from build123d import *

# Parameters (mm, degrees)
F0_W     = 304.8
F0_H     = 381
F1_DEPTH = 355.6
F2_R     = 25.4
F3_R     = 127
F4_DEPTH = 152.4


with BuildPart() as f1:
    # F0 (on Front) → F1 (new body)
    with BuildSketch(Plane.XZ):
        Rectangle(F0_W, F0_H)
    extrude(amount=F1_DEPTH)

    # F2
    f2_edges = [f1.edges().sort_by_distance(p)[0] for p in [
        (-152.4, -355.6, 0),
        (0, -355.6, 190.5),
        (152.4, -355.6, 0),
        (0, -355.6, -190.5),
        (-152.4, -177.8, -190.5),
        (-152.4, -177.8, 190.5),
        (152.4, -177.8, 190.5),
        (152.4, -177.8, -190.5),
        (0, 0, -190.5),
        (152.4, 0, 0),
        (0, 0, 190.5),
        (-152.4, 0, 0),
    ]]
    fillet(f2_edges, radius=F2_R)

    # F3 (on face) → F4 (join)
    with BuildSketch(Plane(origin=(0, 0, 0), x_dir=(-1, 0, 0), z_dir=(0, 1, 0))):
        Circle(F3_R)
    extrude(amount=F4_DEPTH)


solid = f1.part
The model under review builds one solid part; all positions refer to its coordinate system, in mm. A direction names the side the tool comes from. Coordinates: 2 decimals unless noted, no trailing zeros. Write each loop counter-clockwise with the first axis right and the second up, starting at its lowest first coordinate (ties: lowest second). Pieces come first, ordered by that corner, then holes. Notation, with made-up numbers: M 20,67 L 77,67 A22 ccw 77,93 Z; hole C -8.75,58 d8. An arc over 180 degrees is marked long. Put each result on its own line as item: value.
1) Wall thickness on probe 1 along Y at (x, z) = (-57, -135); probe 2 along Z at (x, y) = (-129, -49); probe 3 along X at (y, z) = (-226, -167): over which ranges is each line inside the solid? List them lowest first. Write a range as [from, to].
Computed:
probe 1: y = [-355.6, 0]
probe 2: z = [-190.42, 190.42]
probe 3: x = [-152.33, 152.33]
2) Clearance check with a flat-ended pin moving along its axis: pin 1 Ø2 at (x, z) = (31, 131.5) entering from +Y. State where the tip first meets the part, or that it passes through.
Computed:
pin 1: stops at y = 0
3) Add section A-A on x = 0. Give the boundary of the cut face in (y, z).
Computed:
outline: M -355.6,-165.1 A25.4 ccw -330.2,-190.5 L -25.4,-190.5 A25.4 ccw 0,-165.1 L 0,-127 L 152.4,-127 L 152.4,127 L 0,127 L 0,165.1 A25.4 ccw -25.4,190.5 L -330.2,190.5 A25.4 ccw -355.6,165.1 Z
4) For faces 1 (the flat face through (152.4, -176, -2)), 2 (the cylindrical face through (27.53, 75.13, -123.98)), 3 (the flat face through (-2, 0, -136)), list the 3-axis set-ups (+Z, -Z, +X, -X, +Y, -Y) from which the entire face can be reached by the end or side of a thin tool; tool diameter is ignored.
Computed:
face 1: +Z, -Z, +X, +Y, -Y
face 2: +Y
face 3: -Z, +Y
5) Add section B-B on z = -33. Give the boundary of the cut face in (x, y), then the cut area to 3 significant figures.
Computed:
outline: M -152.4,-330.2 A25.4 ccw -127,-355.6 L 127,-355.6 A25.4 ccw 152.4,-330.2 L 152.4,-25.4 A25.4 ccw 127,0 L 122.64,0 L 122.64,152.4 L -122.64,152.4 L -122.64,0 L -127,0 A25.4 ccw -152.4,-25.4 Z
area: 145,000 mm2
6) Add section C-C on y = 42.5. Give the boundary of the cut face in (x, z).
Computed:
outline: C 0,0 d254
